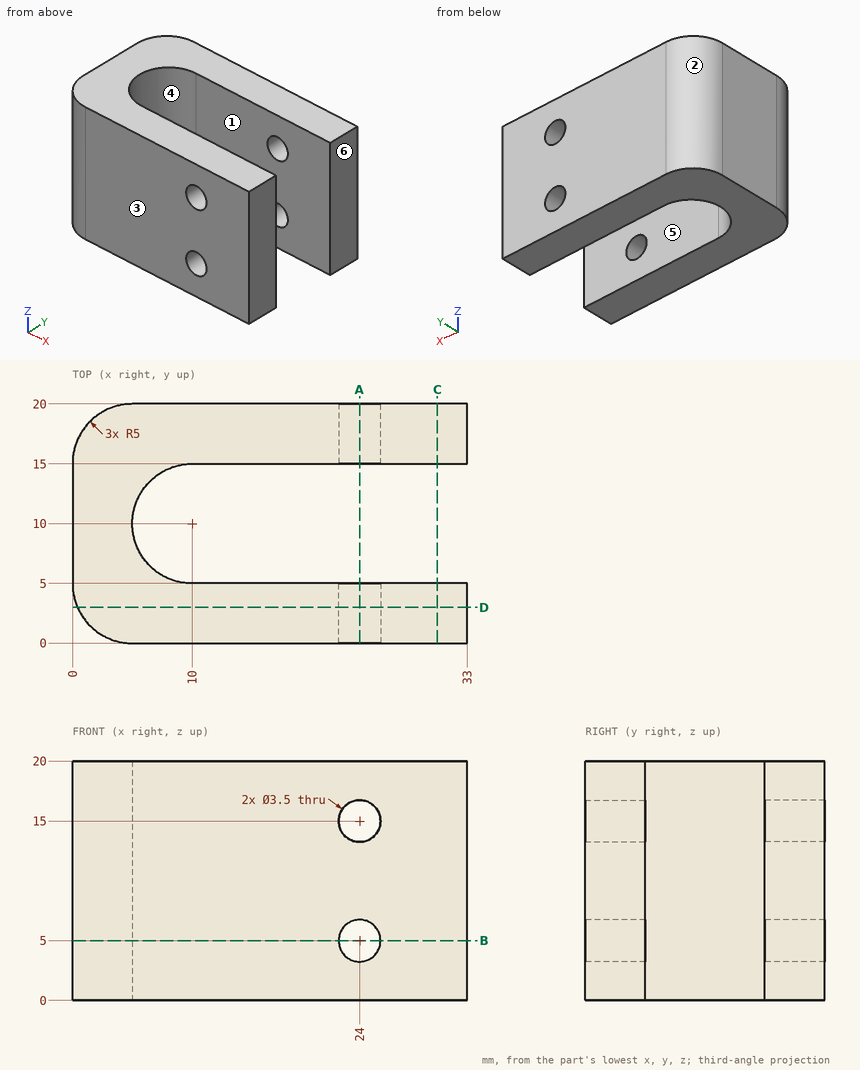
For this review, use the dimensioned drawing (mm, ordinates from the lowest corner) and the shaded views. A direction names the side the tool comes from. Give positions to 0.01 mm unless a question says otherwise; leave off trailing zeros. Order: outer loops, then holes, each group sorted by start corner. A loop starts at its lowest first (then second) coordinate and runs counter-clockwise, first axis right, second up. Notation, with made-up numbers: (47, 12) - (63, 12) arc R23 cw to (63, 20) - close; hole circle Ø9 at (11, -16.75). An arc over 180 degrees is marked (long way). Write item = value, one per line. Start each with the question number.
Q1. We need section D-D on y = 3. State the section outline as (x, z) points.
Q2. We need section C-C on x = 30.5. State the section outline as (y, z) points.
Q3. Clearance check with flat-ended pins moving along their axes: pin 1 Ø1.5 at (y, z) = (2.5, 6.5) entering from -X; pin 2 Ø3 at (x, z) = (24, 15) entering from +Y. State where each tip first meets the part, or that it passes through.
Q4. Tool access review of the marked faces 1 and 2: name each direction out of +Z, -Z, +X, -X, +Y, -Y from which nothing blocks a thin tool from reaching the whole face with its end or side.
Q5. To check wall thickness, follow L1, parallel to Z at x = 24, y = 2.6; L2, parallel to Y at x = 18, z = 8; L3, parallel to Y at x = 8.5, z = 15.75. State the ranges of each line that lie inside material, in increasing order. Write a range as from..to.
Q6. Mouldability with a two-part tool opening along Y and no side actions: class the marked faces 3, 4, 5 and 6 as released by +Y, released by -Y, zero draft, split by the parting line, or undercut.
Q7. We need section A-A on x = 24. State the section outline as (y, z) points, plus the area to 3 significant figures.
Q8. We need section B-B on z = 5. State the section outline as (x, y) points.
Working result:
q1.outline = (0.42, 0) - (33, 0) - (33, 20) - (0.42, 20) - close; hole circle Ø3.5 at (24, 5); hole circle Ø3.5 at (24, 15)
q2.outline = (0, 0) - (5, 0) - (5, 20) - (0, 20) - close; (15, 0) - (20, 0) - (20, 20) - (15, 20) - close
q3.pin_1 = 0.32
q3.pin_2 = through
q4.face_1 = +Z, -Z, +X
q4.face_2 = +Z, -Z, -X, +Y
q5.L1 = 0..3.25, 6.75..13.25, 16.75..20
q5.L2 = 0..5, 15..20
q5.L3 = 0..5.23, 14.77..20
q6.face_3 = released by -Y
q6.face_4 = undercut
q6.face_5 = undercut
q6.face_6 = zero draft
q7.outline = (0, 0) - (5, 0) - (5, 3.25) - (0, 3.25) - close; (0, 6.75) - (5, 6.75) - (5, 13.25) - (0, 13.25) - close; (0, 16.75) - (5, 16.75) - (5, 20) - (0, 20) - close; (15, 0) - (20, 0) - (20, 3.25) - (15, 3.25) - close; (15, 6.75) - (20, 6.75) - (20, 13.25) - (15, 13.25) - close; (15, 16.75) - (20, 16.75) - (20, 20) - (15, 20) - close
q7.area = 130 mm²
q8.outline = (0, 5) arc R5 ccw to (5, 0) - (22.25, 0) - (22.25, 5) - (10, 5) arc R5 cw to (10, 15) - (22.25, 15) - (22.25, 20) - (5, 20) arc R5 ccw to (0, 15) - close; (25.75, 0) - (33, 0) - (33, 5) - (25.75, 5) - close; (25.75, 15) - (33, 15) - (33, 20) - (25.75, 20) - close
